```python
from build123d import *

# Parameters (mm, degrees)
F0_R     = 2.54
F0_R_2   = 4.191
F0_R_3   = 14.2875
F0_R_4   = 4.7625
F1_DEPTH = 3.175


with BuildPart() as f1:
    # F0 (on Front) → F1 (new body)
    with BuildSketch(Plane.XZ):
        with BuildLine():
            ThreePointArc((0, 6.35), (1.859872, 1.859872), (6.35, 0))
            Line((6.35, 0), (98.425, 0))
            ThreePointArc((98.425, 0), (102.915128, 1.859872), (104.775, 6.35))
            Line((104.775, 6.35), (104.775, 57.15))
            ThreePointArc((104.775, 57.15), (102.915128, 61.640128), (98.425, 63.5))
            Line((98.425, 63.5), (6.35, 63.5))
            ThreePointArc((6.35, 63.5), (1.859872, 61.640128), (0, 57.15))
            Line((0, 57.15), (0, 6.35))
        make_face()
        with Locations((6.35, 6.35)):
            Circle(F0_R, mode=Mode.SUBTRACT)
        with Locations((73.025, 6.35)):
            Circle(F0_R_2, mode=Mode.SUBTRACT)
        with Locations((98.425, 6.35)):
            Circle(F0_R, mode=Mode.SUBTRACT)
        with Locations((32.3342, 31.75)):
            Circle(F0_R_3, mode=Mode.SUBTRACT)
        with Locations((6.35, 57.15)):
            Circle(F0_R, mode=Mode.SUBTRACT)
        with Locations((73.025, 31.75)):
            Circle(F0_R_4, mode=Mode.SUBTRACT)
        with Locations((73.025, 57.15)):
            Circle(F0_R_2, mode=Mode.SUBTRACT)
        with Locations((98.425, 57.15)):
            Circle(F0_R, mode=Mode.SUBTRACT)
    extrude(amount=F1_DEPTH)


solid = f1.part
```
The model under review builds one solid part; all positions refer to its coordinate system, in mm. Coordinates: 2 decimals unless noted, no trailing zeros. Write each loop counter-clockwise with the first axis right and the second up, starting at its lowest first coordinate (ties: lowest second). Pieces come first, ordered by that corner, then holes. Notation, with made-up numbers: (49.5, 15) -> (92.5, 15) arc R29 ccw to (92.5, 52) -> close; hole circle Ø9 at (58.25, -10.5). An arc over 180 degrees is marked (long way). One line per item, written item: value. Start each with the question number.
Q1. Add section B-B, the plane y = -2.3. Count the separate pieces of the cut face and the enclosed holes in it, then the cut area to 3 significant figures.
Q2. Add section D-D, the plane z = 22. Give the boundary of the cut face in (x, y) (3 decimals).
Q3. Add section C-C, the plane x = 39. Give the boundary of the cut face in (y, z) (3 decimals).
Q4. Add section A-A, the plane z = 31.75. Give the boundary of the cut face in (x, y) (1 decimal).
Q5. Clearance check with a flat-ended pin moving along its axis: P1, Ø5, axis at x = 24, z = 37, coming from the -Y side. State where the tip first meets the part, or that it passes through.
Q6. The part is to be moulded in two halves that separate along Z. For faces 1 (the face through (53, -2, 63.5)), 2 (the face through (20.996, -1.565, 23.056)), 3 (the face through (96.409, -1.565, 55.604)), 4 (the face through (1.81, -1.57, 1.91)), say which applies: +Z half, -Z half, draft (parallel to the pull), parting line (faces both ways), or undercut.
Q7. To check wall thickness, follow probe 1 along Z at (x, y) = (6.5, -1.5); probe 2 along X at (y, z) = (-0.8, 8) (3 decimals); probe 3 along X at (y, z) = (-0.55, 36) (3 decimals). State the ranges of each line that lie inside material, in increasing order.
Response:
1. separate pieces: 1
1. enclosed holes: 8
1. area: 5,710 mm²
2. outline: (0, -3.175) -> (21.891, -3.175) -> (21.891, 0) -> (0, 0) -> close; (42.778, -3.175) -> (104.775, -3.175) -> (104.775, 0) -> (42.778, 0) -> close
3. outline: (-3.175, 0) -> (0, 0) -> (0, 19.113) -> (-3.175, 19.113) -> close; (-3.175, 44.387) -> (0, 44.387) -> (0, 63.5) -> (-3.175, 63.5) -> close
4. outline: (0, -3.2) -> (18, -3.2) -> (18, 0) -> (0, 0) -> close; (46.6, -3.2) -> (68.3, -3.2) -> (68.3, 0) -> (46.6, 0) -> close; (77.8, -3.2) -> (104.8, -3.2) -> (104.8, 0) -> (77.8, 0) -> close
5. P1: through
6. face 1: +Z half
6. face 2: undercut
6. face 3: undercut
6. face 4: -Z half
7. probe 1: 0 to 3.81, 8.89 to 54.61, 59.69 to 63.5
7. probe 2: 0 to 4.419, 8.281 to 69.172, 76.878 to 96.494, 100.356 to 104.775
7. probe 3: 0 to 18.693, 45.975 to 70.876, 75.174 to 104.775
